Build history of the part. All positions in model axes, mm. A direction names the side the tool comes from. Coordinates: 2 decimals unless noted, no trailing zeros. Write each loop counter-clockwise with the first axis right and the second up, starting at its lowest first coordinate (ties: lowest second). Pieces come first, ordered by that corner, then holes.
Autodesk Fusion 360 part; units mm, degrees
sketch "Sketch4" plane through (0, 11.5, 0) normal (0, 1, 0) x (-1, 0, 0) in component "Plunger"
  circle A0 centre (0, 0) radius 3.25
  circle A1 centre (0, 0) radius 6.5
  circle A2 centre (0, 0) radius 10.75
  dimension "d20" = 13
  dimension "d21" = 21.5
extrude "Extrude3" add sketch "Sketch4" against normal blind 3 contours A2 in component "Plunger"
sketch "Sketch5" plane through (0, 11.5, 0) normal (0, 1, 0) x (-1, 0, 0) in component "Plunger"
  circle A0 centre (0, 0) radius 6.5
  circle A1 centre (0, 0) radius 10.75
  circle A2 centre (0, 0) radius 9.15
extrude "Extrude4" add sketch "Sketch5" along normal blind 6 contours A0 | A1 | A2 in component "Plunger"
sketch "Sketch1" plane through (0, 11.5, 0) normal (0, -1, 0) x (1, 0, 0)
  circle A0 centre (0, 0) radius 6.5
  circle A1 centre (0, 0) radius 3.25
  dimension "d29" = 6.5
extrude "Extrude6" cut sketch "Sketch1" against normal blind 3.5 contours A1 in component "Plunger"
sketch "Sketch7" plane through (0, 17.5, 0) normal (0, 1, 0) x (-1, 0, 0) in component "Plunger"
  circle A0 centre (0, 0) radius 10.75
  line L0 (4.0415, -7) -> (8.0829, 0)
  line L1 (8.0829, 0) -> (4.0415, 7)
  line L2 (4.0415, 7) -> (-4.0415, 7)
  line L3 (-4.0415, 7) -> (-8.0829, 0)
  line L4 (-8.0829, 0) -> (-4.0415, -7)
  line L5 (-4.0415, -7) -> (4.0415, -7)
  dimension "d32" = 7
extrude "Extrude7" add sketch "Sketch7" along normal blind 6.5 in component "Plunger"
fillet "Fillet1" radius 1 1 edges at (6.0601, 8.5, -2.3505) in component "Plunger"
fillet "Fillet2" radius 1 1 edges at (10.0225, 8.5, 3.8874) in component "Plunger"
fillet "Fillet3" radius 1 1 edges at (10.0225, 24, -3.8874) in component "Plunger"
component "Plunger" placed x (1, 0, 0) y (0, 1, 0) z (0, 0, 1) at (0, 0, 0)
1. Probe line 1 along Z through (x, y) = (0, 9.9); line 2 along Y through (x, z) = (1.5, -2); line 3 along Z through (x, y) = (0, 12.6). List the from-to ranges inside material, lowest first.
Computed values:
line 1: z = -10.75 to -6.5, 6.5 to 10.75
line 2: y = 15 to 17.5
line 3: z = -10.75 to -3.25, 3.25 to 10.75
2. Saw through at C-C on y = 12. List the corners of the cut face in (x, z), plus the area to 3 significant figures.
Computed values:
outline: circle Ø21.5 at (0, 0); hole circle Ø6.5 at (0, 0)
area: 330 mm2
3. Mould opens along Z. For faces 4 (the face through (1.4, 16.16, -10.66)), 5 (the face through (6.09, 20.7, -3.45)), 6 (the face through (-0.7, 24, -7.2)), 7 (the face through (0, 21, -7)) say: +Z half, -Z half, draft (parallel to the pull), parting line (faces both ways), or undercut.
Computed values:
face 4: parting line
face 5: undercut
face 6: draft
face 7: undercut
4. 3-axis set-ups, long thin cutter, end or side, ignore diameter. For faces 1 (the face through (5.158, 10.514, -3.955)), 2 (the face through (-5, 8.5, -6)), 3 (the face through (-6.034, 20.704, -3.549)): which of +Z, -Z, +X, -X, +Y, -Y reach the whole face in a straight line?
Computed values:
face 1: -Y
face 2: +Z, -Z, +X, -X, -Y
face 3: +Y
5. Saw through at A-A on y = 20.25. List the corners of the cut face in (x, z), plus the area to 3 significant figures.
Computed values:
outline: circle Ø21.5 at (0, 0); hole (-8.08, 0) - (-4.04, -7) - (4.04, -7) - (8.08, 0) - (4.04, 7) - (-4.04, 7) - close
area: 193 mm2
6. Saw through at B-B on x = 0. List the corners of the cut face in (y, z), plus the area to 3 significant figures.
Computed values:
outline: (8.5, -9.75) arc R1 ccw to (9.5, -10.75) - (23, -10.75) arc R1 ccw to (24, -9.75) - (24, -7) - (17.5, -7) - (17.5, 7) - (24, 7) - (24, 9.75) arc R1 ccw to (23, 10.75) - (9.5, 10.75) arc R1 ccw to (8.5, 9.75) - (8.5, 7.5) arc R1 ccw to (9.5, 6.5) - (11.5, 6.5) - (11.5, 3.25) - (15, 3.25) - (15, -3.25) - (11.5, -3.25) - (11.5, -6.5) - (9.5, -6.5) arc R1 ccw to (8.5, -7.5) - close
area: 179 mm2
7. Flat gauge pins, fed straight in: pin 1 (5 mm diameter, centred on x = 0, z = 1.5, fed in from -Y); pin 2 (2 mm diameter, centred on x = 4.5, y = 16, fed in from -Z); pin 3 (5 mm diameter, centred on x = 0, z = 0, fed in from +Y). Where does each tip first touch, or does it go through?
Computed values:
pin 1: stops at y = 11.5
pin 2: stops at z = -10.16
pin 3: stops at y = 17.5
